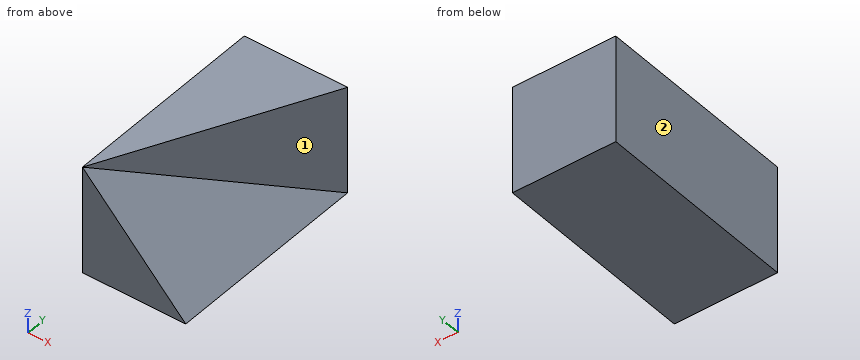
```python
from build123d import *

# Parameters (mm, degrees)
F1_DEPTH = 52
F3_DEPTH = 100


# Not quite as in the source:
# - an extrude ends at something that could not be found from the text; its depth is read off the source's solid


with BuildPart() as f1:
    # F0 (on Top) → F1 (new body)
    with BuildSketch(Plane.XY):
        Polygon((0, 100), (0, 0), (50, 100), align=None)
    extrude(amount=F1_DEPTH)

    # F2 (on face) → F3 (join, through all)
    with BuildSketch(Plane(origin=(0, 100, 0), x_dir=(-1, 0, 0), z_dir=(0, 1, 0))):
        Polygon((0, 52), (-50, 0), (0, 0), align=None)
    extrude(amount=-F3_DEPTH)


solid = f1.part
```
Read the model definition and answer for the solid it produces. Units are mm, in the model's axes. Face numbers are marked on the shaded views. A direction names the side the tool comes from. Give positions to 0.01 mm unless a question says otherwise; leave off trailing zeros. Loops run counter-clockwise (first coordinate to the right, second up) from the corner with the lowest first, then second, coordinate; pieces in that order, holes last.
Item 1: For the marked faces 1 and 2, determine the directions among +Z, -Z, +X, -X, +Y, -Y from which every point of the face is accessible in a straight line to the end or side of a thin tool.
Item 2: The part is cut by section B-B (x = 10.5). Write down the section's boundary in (y, z).
Item 3: Each of these flat-tipped pins is pushed along its axis until it touches: pin 1 Ø2 at (x, y) = (24.5, 14.5) entering from +Z; pin 2 Ø10 at (y, z) = (84.5, 42) entering from +X. Where does it stop, or does it pass through?
Item 4: Find the intervals of material crossed by line 1 along X through (y, z) = (30.5, 47); line 2 along Y through (x, z) = (45.5, 23); line 3 along X through (y, z) = (41.5, 34), in increasing order.
Item 5: The part is cut by section D-D (x = 16.5). Write down the section's boundary in (y, z), and give its area (3 significant figures).
Item 6: The part is cut by section C-C (z = 11). Write down the section's boundary in (x, y).
Item 7: The part is cut by section A-A (y = 23). Write down the section's boundary in (x, z).
Taken from the geometry:
1. face 1: +Z, +X, -Y
1. face 2: +Z, -Z, -X, +Y, -Y
2. outline: (0, 0) - (100, 0) - (100, 52) - (21, 52) - (21, 41.08) - (0, 41.08) - close
3. pin 1: stops at z = 27.56
3. pin 2: stops at x = 44.75
4. line 1: x = 0 to 15.25
4. line 2: y = 91 to 100
4. line 3: x = 0 to 20.75
5. outline: (0, 0) - (100, 0) - (100, 52) - (33, 52) - (33, 34.84) - (0, 34.84) - close
5. area: 4,630 mm2
6. outline: (0, 0) - (39.42, 0) - (39.42, 78.85) - (50, 100) - (0, 100) - close
7. outline: (0, 0) - (50, 0) - (11.5, 40.04) - (11.5, 52) - (0, 52) - close
